Check sheet for the modelled part. Datum: model origin and axes. Units: mm. Face numbers are marked on the shaded views. A direction names the side the tool comes from. Give positions to 0.01 mm unless a question says otherwise; leave off trailing zeros. Order: outer loops, then holes, each group sorted by start corner. A loop starts at its lowest first (then second) coordinate and runs counter-clockwise, first axis right, second up.
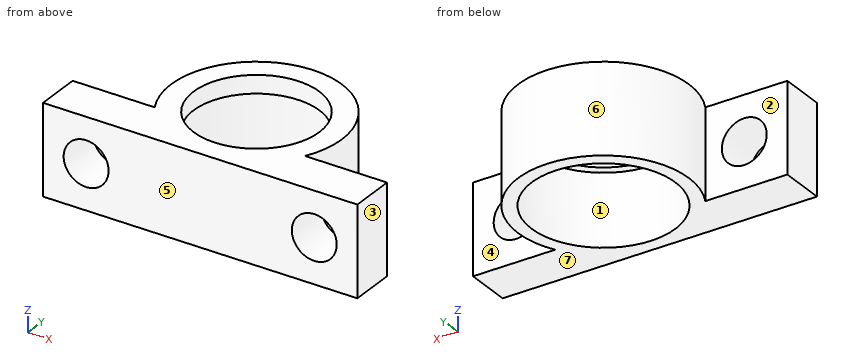
```python
from build123d import *

# Parameters (mm, degrees)
F0_R     = 8
F1_DEPTH = 8
F3_DEPTH = 2
F4_R     = 2.5
F5_DEPTH = 25.4


with BuildPart() as f1:
    # F0 (on Top) → F1 (new body)
    with BuildSketch(Plane.XY):
        with BuildLine():
            Line((17.5, -4.5), (8.3666, -4.5))
            ThreePointArc((8.3666, -4.5), (0, 9.5), (-8.3666, -4.5))
            Line((-8.3666, -4.5), (-17.5, -4.5))
            Line((-17.5, -4.5), (-17.5, -9.5))
            Line((-17.5, -9.5), (0, -9.5))
            Line((0, -9.5), (17.5, -9.5))
            Line((17.5, -9.5), (17.5, -4.5))
        make_face()
        Circle(F0_R, mode=Mode.SUBTRACT)
    extrude(amount=-F1_DEPTH)

    # F2 (on Top) + F0 (on Top) → F3 (join)
    with BuildSketch(Plane.XY):
        with BuildLine():
            ThreePointArc((0, -7), (4.949747, -4.949747), (7, 0))
            ThreePointArc((7, 0), (-4.949747, 4.949747), (0, -7))
        make_face()
        with BuildLine():
            Line((17.5, -4.5), (8.3666, -4.5))
            ThreePointArc((8.3666, -4.5), (0, 9.5), (-8.3666, -4.5))
            Line((-8.3666, -4.5), (-17.5, -4.5))
            Line((-17.5, -4.5), (-17.5, -9.5))
            Line((-17.5, -9.5), (0, -9.5))
            Line((0, -9.5), (17.5, -9.5))
            Line((17.5, -9.5), (17.5, -4.5))
        make_face()
        with BuildLine():
            ThreePointArc((0, -7), (-4.949747, 4.949747), (7, 0))
            ThreePointArc((7, 0), (4.949747, -4.949747), (0, -7))
        make_face(mode=Mode.SUBTRACT)
    with BuildSketch(Plane.XY):
        with BuildLine():
            Line((17.5, -4.5), (8.3666, -4.5))
            ThreePointArc((8.3666, -4.5), (0, 9.5), (-8.3666, -4.5))
            Line((-8.3666, -4.5), (-17.5, -4.5))
            Line((-17.5, -4.5), (-17.5, -9.5))
            Line((-17.5, -9.5), (0, -9.5))
            Line((0, -9.5), (17.5, -9.5))
            Line((17.5, -9.5), (17.5, -4.5))
        make_face()
        Circle(F0_R, mode=Mode.SUBTRACT)
    extrude(amount=F3_DEPTH)

    # F4 (on face) → F5 (cut)
    with BuildSketch(Plane.XZ.offset(9.5)):
        with Locations((-12.7, -3)):
            Circle(F4_R)
        with Locations((12.7, -3)):
            Circle(F4_R)
    extrude(amount=-F5_DEPTH, mode=Mode.SUBTRACT)


solid = f1.part
```
Q1. Tool access check on the marked faces 1, 2, 3 and 4. Record the directions out of +Z, -Z, +X, -X, +Y, -Y that give a thin tool (end or side, any length) a straight path to the whole face; none if there is none.
Q2. Sectioned sample at A-A, the plane z = -3. Record the cut outline in (x, y), plus the area to 3 significant figures.
Q3. Sectioned sample at D-D, the plane y = -2.25. Record the cut outline in (x, z), plus the area to 3 significant figures.
Q4. Draft check along Y on the marked faces 5, 6 and 7. Enter one of: pulls with the +Y half, pulls with the -Y half, needs draft (parallel to the pull), parting line crosses it, or undercut.
Q5. Go/stop test with flat-tipped pins: P1, Ø4.5, axis at x = -11, z = -1.5, coming from the +Y side; P2, Ø5, axis at x = -2, y = -2.5, coming from the -Z side; P3, Ø4.5, axis at x = 12, z = -5, coming from the +Y side; P4, Ø6, axis at x = 7, z = -1, coming from the +Y side. Record where each tip stops, or that it passes through.
Q6. Sectioned sample at C-C, the plane z = -7. Record the cut outline in (x, y).
Q7. Sectioned sample at B-B, the plane x = 12.7. Record the cut outline in (y, z).
Q8. Material ranges on line 1 (Z direction, x = -12.7, y = -7.35); line 2 (X direction, y = -6.25, z = -1.75); line 3 (X direction, y = -8.25, z = -0.75), recorded low to high.
Filled in:
1. face 1: -Z
1. face 2: +Z, -Z, -X
1. face 3: +Z, -Z, +X, +Y, -Y
1. face 4: +Z, -Z, +X
2. outline: (-17.5, -9.5) - (-15.2, -9.5) - (-15.2, -4.5) - (-17.5, -4.5) - close; (-10.2, -9.5) - (10.2, -9.5) - (10.2, -4.5) - (8.37, -4.5) arc R9.5 ccw (long way) to (-8.37, -4.5) - (-10.2, -4.5) - close; (15.2, -9.5) - (17.5, -9.5) - (17.5, -4.5) - (15.2, -4.5) - close; hole circle Ø16 at (0, 0)
2. area: 148 mm2
3. outline: (-9.23, -8) - (-7.68, -8) - (-7.68, 0) - (-6.63, 0) - (-6.63, 2) - (-9.23, 2) - close; (6.63, 0) - (7.68, 0) - (7.68, -8) - (9.23, -8) - (9.23, 2) - (6.63, 2) - close
3. area: 35.2 mm2
4. face 5: pulls with the -Y half
4. face 6: undercut
4. face 7: needs draft
5. P1: stops at y = 3.7
5. P2: passes through
5. P3: stops at y = -4.5
5. P4: stops at y = 8.62
6. outline: (-17.5, -9.5) - (17.5, -9.5) - (17.5, -4.5) - (8.37, -4.5) arc R9.5 ccw (long way) to (-8.37, -4.5) - (-17.5, -4.5) - close; hole circle Ø16 at (0, 0)
7. outline: (-9.5, -8) - (-4.5, -8) - (-4.5, -5.5) - (-9.5, -5.5) - close; (-9.5, -0.5) - (-4.5, -0.5) - (-4.5, 2) - (-9.5, 2) - close
8. line 1: z = -8 to -5.5, -0.5 to 2
8. line 2: x = -17.5 to -14.87, -10.53 to -4.99, 4.99 to 10.53, 14.87 to 17.5
8. line 3: x = -17.5 to -13.79, -11.61 to 11.61, 13.79 to 17.5
